Here's how the part is built. I have some questions about the finished solid (model axes, mm). Face numbers are marked on the shaded views. Round coordinates to 2 decimals unless told otherwise and drop trailing zeros. Write each loop counter-clockwise with the first axis right and the second up, starting at its lowest first coordinate (ties: lowest second). Pieces come first, ordered by that corner, then holes. Notation, with made-up numbers: (26.25, -30) -> (61.25, -30) arc R13 ccw to (61.25, -8) -> close; hole circle Ø2 at (44, 22.5). An arc over 180 degrees is marked (long way). Answer in a Markdown table with one row per item.
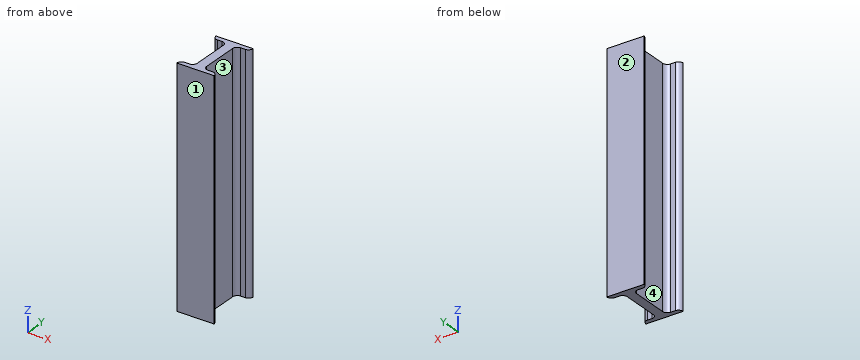
from build123d import *

# Parameters (mm, degrees)
DODANIE_WYCI_GNI_CIE1_DEPTH = 250
ZAOKR_GLENIE2_DEPTH         = 250
ZAOKR_GLENIE2_2_DEPTH       = 250


with BuildPart() as part:
    # Szkic1 → Dodanie-wyciągnięcie1 (new body)
    with BuildSketch(Plane.XY):
        Polygon((0, 0), (40, 0), (40, 5), (25, 5), (25, 55), (40, 55), (40, 60), (0, 60), (0, 55), (15, 55), (15, 5), (0, 5), align=None)
    extrude(amount=DODANIE_WYCI_GNI_CIE1_DEPTH)

    # Zaokrąglenie2: read off the stored shape, not the designer's step
    # Zaokrąglenie2 outline → Zaokrąglenie2 (cut)
    with BuildSketch(Plane.XY):
        with BuildLine():
            Line((40, 55), (40, 60))
            ThreePointArc((40, 60), (38.535533906, 56.464466094), (35, 55))
            Line((35, 55), (40, 55))
        make_face()
        with BuildLine():
            Line((40, 5), (35, 5))
            ThreePointArc((35, 5), (38.535533906, 3.535533906), (40, 0))
            Line((40, 0), (40, 5))
        make_face()
        with BuildLine():
            Line((0, 55), (5, 55))
            ThreePointArc((5, 55), (1.464466094, 56.464466094), (0, 60))
            Line((0, 60), (0, 55))
        make_face()
        with BuildLine():
            ThreePointArc((0, 0), (1.464466094, 3.535533906), (5, 5))
            Line((5, 5), (0, 5))
            Line((0, 5), (0, 0))
        make_face()
    extrude(amount=ZAOKR_GLENIE2_DEPTH, mode=Mode.SUBTRACT)

    # Zaokr_glenie2 2 outline → Zaokr_glenie2 2 (add)
    with BuildSketch(Plane.XY):
        with BuildLine():
            ThreePointArc((30, 5), (26.464466094, 6.464466094), (25, 10))
            Line((25, 10), (25, 5))
            Line((25, 5), (30, 5))
        make_face()
        with BuildLine():
            ThreePointArc((25, 50), (26.464466094, 53.535533906), (30, 55))
            Line((30, 55), (25, 55))
            Line((25, 55), (25, 50))
        make_face()
        with BuildLine():
            ThreePointArc((10, 55), (13.535533906, 53.535533906), (15, 50))
            Line((15, 50), (15, 55))
            Line((15, 55), (10, 55))
        make_face()
        with BuildLine():
            ThreePointArc((15, 10), (13.535533906, 6.464466094), (10, 5))
            Line((10, 5), (15, 5))
            Line((15, 5), (15, 10))
        make_face()
    extrude(amount=ZAOKR_GLENIE2_2_DEPTH)


solid = part.part
1) I want a section at A-A, the plane z = 105. List the corners of the cut face in (x, y) for me, and give its area (3 significant figures).
Response:
| item | result |
|---|---|
| outline | (0, 0) -> (40, 0) arc R5 ccw to (35, 5) -> (30, 5) arc R5 cw to (25, 10) -> (25, 50) arc R5 cw to (30, 55) -> (35, 55) arc R5 ccw to (40, 60) -> (0, 60) arc R5 ccw to (5, 55) -> (10, 55) arc R5 cw to (15, 50) -> (15, 10) arc R5 cw to (10, 5) -> (5, 5) arc R5 ccw to start |
| area | 900 mm^2 |
2) We'd pull the mould along Y, two halves only. Please class the marked faces 1, 2, 3 and 4: +Y half, -Y half, draft (parallel to the pull), parting line (faces both ways), or undercut.
Response:
| item | result |
|---|---|
| face 1 | -Y half |
| face 2 | +Y half |
| face 3 | undercut |
| face 4 | undercut |
3) I want a section at B-B, the plane y = 18. List the corners of the cut face in (x, z) for me, and give its area (3 significant figures).
Response:
| item | result |
|---|---|
| outline | (15, 0) -> (25, 0) -> (25, 250) -> (15, 250) -> close |
| area | 2,500 mm^2 |
4) I need wall thicknesses on line 1 (Y direction, x = 31, z = 92); line 2 (X direction, y = 42, z = 116.5); line 3 (X direction, y = 3, z = 122). Which ranges of each line are inside material? Lowest first, please. Write a range as [from, to].
Response:
| item | result |
|---|---|
| line 1 | y = [0, 5], [55, 60] |
| line 2 | x = [15, 25] |
| line 3 | x = [1, 39] |
5) For pin 1 (8 mm diameter, centred on x = 9.5, y = 42.5, fed in from +Z); pin 2 (1.5 mm diameter, centred on y = 39.5, z = 181.5, fed in from +X); pin 3 (12 mm diameter, centred on y = 18, z = 155, fed in from -X); pin 4 (2 mm diameter, centred on y = 9.5, z = 77.5, fed in from +X), each with a flat end and sliding along its axis, tell me the tip position at first contact or that it passes through.
Response:
| item | result |
|---|---|
| pin 1 | passes through |
| pin 2 | stops at x = 25 |
| pin 3 | stops at x = 15 |
| pin 4 | stops at x = 25.23 |
